Source: three-view drawing plus pictorial views. Frame: mm from the lowest corner of the part. A direction names the side the tool comes from. Round coordinates to 2 decimals unless told otherwise and drop trailing zeros. Order: outer loops, then holes, each group sorted by start corner. A loop starts at its lowest first (then second) coordinate and runs counter-clockwise, first axis right, second up. Notation, with made-up numbers: (-30.75, 19) -> (-19.75, 19) arc R14 ccw to (-19.75, 34) -> close; hole circle Ø7 at (36, 81.5). An arc over 180 degrees is marked (long way). Use a Markdown table: item, result.
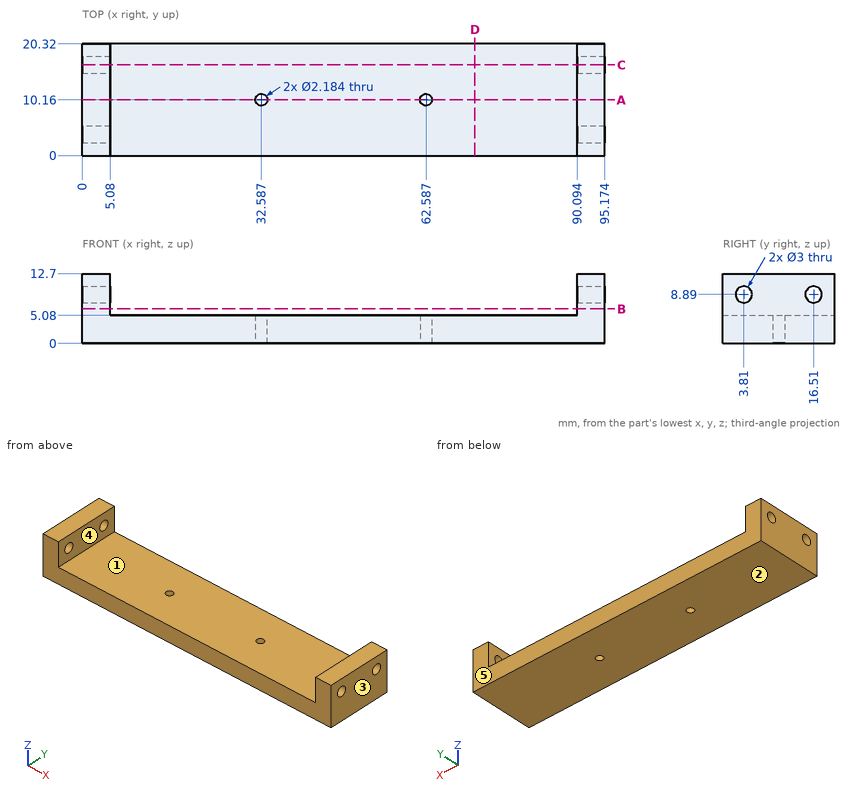
1) Cut plane B-B on z = 6.25. Return loops of the section in (x, y).
Results found:
| item | result |
|---|---|
| outline | (0, 0) -> (5.08, 0) -> (5.08, 20.32) -> (0, 20.32) -> close; (90.09, 0) -> (95.17, 0) -> (95.17, 20.32) -> (90.09, 20.32) -> close |
2) Pin query (flat end, axial travel): pin 1 Ø5 at (x, y) = (21, 2) entering from +Z; pin 2 Ø1.7 at (x, y) = (32.59, 10.16) entering from -Z. Return the tip coordinate at first contact, or that it passes through.
Results found:
| item | result |
|---|---|
| pin 1 | stops at z = 5.08 |
| pin 2 | passes through |
3) Cut plane C-C on y = 16.51. Return loops of the section in (x, z).
Results found:
| item | result |
|---|---|
| outline | (0, 0) -> (95.17, 0) -> (95.17, 7.39) -> (90.09, 7.39) -> (90.09, 5.08) -> (5.08, 5.08) -> (5.08, 7.39) -> (0, 7.39) -> close; (0, 10.39) -> (5.08, 10.39) -> (5.08, 12.7) -> (0, 12.7) -> close; (90.09, 10.39) -> (95.17, 10.39) -> (95.17, 12.7) -> (90.09, 12.7) -> close |
4) Pull-direction query (X, two-part tool) for the marked faces 3, 4 and 5; classes: +X half, -X half, draft (parallel to the pull), parting line (faces both ways), or undercut.
Results found:
| item | result |
|---|---|
| face 3 | +X half |
| face 4 | undercut |
| face 5 | draft |
5) Cut plane A-A on y = 10.16. Return loops of the section in (x, z) (1 decimal).
Results found:
| item | result |
|---|---|
| outline | (0, 0) -> (31.5, 0) -> (31.5, 5.1) -> (5.1, 5.1) -> (5.1, 12.7) -> (0, 12.7) -> close; (33.7, 0) -> (61.5, 0) -> (61.5, 5.1) -> (33.7, 5.1) -> close; (63.7, 0) -> (95.2, 0) -> (95.2, 12.7) -> (90.1, 12.7) -> (90.1, 5.1) -> (63.7, 5.1) -> close |
6) Set-up query: the marked faces 1 and 2. Return all of +Z, -Z, +X, -X, +Y, -Y with unobstructed straight access to the full face (end or side cutting, diameter ignored); none if empty.
Results found:
| item | result |
|---|---|
| face 1 | +Z, +Y, -Y |
| face 2 | -Z, +X, -X, +Y, -Y |
7) Cut plane D-D on x = 71.5. Return loops of the section in (y, z).
Results found:
| item | result |
|---|---|
| outline | (0, 0) -> (20.32, 0) -> (20.32, 5.08) -> (0, 5.08) -> close |
8) Line query: L1, parallel to Y at x = 91, z = 9; L2, parallel to X at y = 13.25, z = 11; L3, parallel to Z at x = 2.05, y = 16.51. Output: solid intervals per line, ascending. Write a range as [from, to].
Results found:
| item | result |
|---|---|
| L1 | y = [0, 2.31], [5.31, 15.01], [18.01, 20.32] |
| L2 | x = [0, 5.08], [90.09, 95.17] |
| L3 | z = [0, 7.39], [10.39, 12.7] |
